Print and shaded views of the part. All mm, measured from the part's lowest x, y and z. A direction names the side the tool comes from. Round coordinates to 2 decimals unless told otherwise and drop trailing zeros. Loops run counter-clockwise (first coordinate to the right, second up) from the corner with the lowest first, then second, coordinate; pieces in that order, holes last. Notation, with made-up numbers: (-15.5, 85) -> (35.5, 85) arc R23 cw to (35.5, 115) -> close; hole circle Ø3 at (-8, -36). An arc over 180 degrees is marked (long way). Use a Markdown table: item, result.
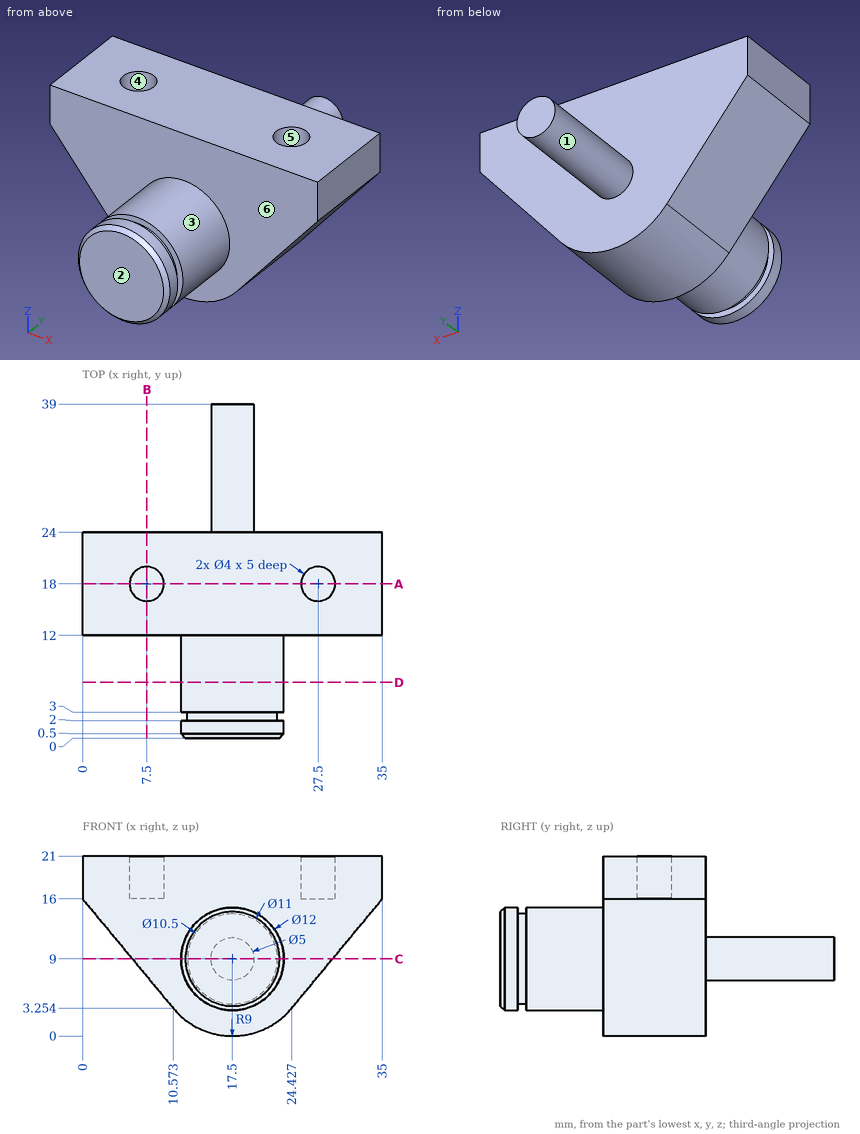
Q1. Band-saw the part on B-B, the plane x = 7.5. Give the cut face in (y, z), plus the area to 4 significant figures.
Results list:
| item | result |
|---|---|
| outline | (12, 6.96) -> (24, 6.96) -> (24, 21) -> (20, 21) -> (20, 16) -> (16, 16) -> (16, 21) -> (12, 21) -> close |
| area | 148.5 mm² |
Q2. Drill centre lines: L1, parallel to Y at x = 27.5, z = 19.25; L2, parallel to Y at x = 13, z = 4.25; L3, parallel to Y at x = 17.5, z = 6.25. Where is each one in solid material? Low to high. Write a range as from..to.
Results list:
| item | result |
|---|---|
| L1 | y = 12..16, 20..24 |
| L2 | y = 12..24 |
| L3 | y = 0..24 |
Q3. Band-saw the part on C-C, the plane z = 9. Give the cut face in (x, y).
Results list:
| item | result |
|---|---|
| outline | (5.81, 12) -> (11.5, 12) -> (11.5, 3) -> (12.25, 3) -> (12.25, 2) -> (11.5, 2) -> (11.5, 0.5) -> (12, 0) -> (23, 0) -> (23.5, 0.5) -> (23.5, 2) -> (22.75, 2) -> (22.75, 3) -> (23.5, 3) -> (23.5, 12) -> (29.19, 12) -> (29.19, 24) -> (20, 24) -> (20, 39) -> (15, 39) -> (15, 24) -> (5.81, 24) -> close |
Q4. Flat gauge pins, fed straight in: pin 1 (6.5 mm diameter, centred on x = 13.5, z = 8.5, fed in from -Y); pin 2 (8 mm diameter, centred on y = 34.5, z = 16, fed in from -X); pin 3 (2 mm diameter, centred on x = 11.5, z = 6, fed in from -Y); pin 4 (3 mm diameter, centred on x = 7.5, y = 18, fed in from +Z). Where does each tip first touch, or does it go through?
Results list:
| item | result |
|---|---|
| pin 1 | stops at y = 0 |
| pin 2 | passes through |
| pin 3 | stops at y = 0.21 |
| pin 4 | stops at z = 16 |
Q5. Band-saw the part on D-D, the plane y = 6.5. Give the cut face in (x, z), plus the area to 3 significant figures.
Results list:
| item | result |
|---|---|
| outline | circle Ø12 at (17.5, 9) |
| area | 113 mm² |
Q6. Tool access for the marked faces 1 and 2: list every direction of +Z, -Z, +X, -X, +Y, -Y with a clear straight run to the whole face (end or side of a thin tool).
Results list:
| item | result |
|---|---|
| face 1 | +Y |
| face 2 | +Z, -Z, +X, -X, -Y |
Q7. Band-saw the part on A-A, the plane y = 18. Give the cut face in (x, z).
Results list:
| item | result |
|---|---|
| outline | (0, 16) -> (10.57, 3.25) arc R9 ccw to (24.43, 3.25) -> (35, 16) -> (35, 21) -> (29.5, 21) -> (29.5, 16) -> (25.5, 16) -> (25.5, 21) -> (9.5, 21) -> (9.5, 16) -> (5.5, 16) -> (5.5, 21) -> (0, 21) -> close |
Q8. Pull direction Y, two halves, no side cores. Call the marked faces 3, 4, 5 and 6: released by +Y, released by -Y, zero draft, split by the parting line, or undercut.
Results list:
| item | result |
|---|---|
| face 3 | zero draft |
| face 4 | undercut |
| face 5 | undercut |
| face 6 | released by -Y |
